from build123d import *

# Parameters (mm, degrees)
F1_DEPTH     = 40.64
F2_SIZE      = 12.7
F3_T1_DEPTH  = 176.0479365306
F3_T3_DEPTH  = 176.0479365306
F3_T5_DEPTH  = 176.0479365306
F3_T7_DEPTH  = 176.0479365306
F3_T9_DEPTH  = 176.0479365306
F3_T11_DEPTH = 176.0479365306
F3_T13_DEPTH = 176.0479365306
F3_T15_DEPTH = 176.0479365306
F3_T17_DEPTH = 176.0479365306
F3_T19_DEPTH = 176.0479365306


# Not quite as in the source:
# - a fillet or chamfer that OpenCascade refuses, or shapes differently, is made with other operations: its cross-section is extruded or revolved along the edge and cut away or added


with BuildPart() as f1:
    # F0 (on Top) → F1 (new body)
    with BuildSketch(Plane.XY):
        Polygon((29.2412366164, 12.8835857291), (16.083875671, 27.6106074452), (-3.2169791099, 31.7913155674), (-21.2890572119, 23.8288216898), (-31.2294390474, 6.7645278386), (-29.2412366164, -12.8835857291), (-16.083875671, -27.6106074452), (3.2169791099, -31.7913155674), (21.2890572119, -23.8288216898), (31.2294390474, -6.7645278386), align=None)
    extrude(amount=F1_DEPTH)

    # F2
    f2_edges = [f1.edges().sort_by_distance(p)[0] for p in [
        (12.253018, -27.810069, 40.64),
        (26.259248, -15.296675, 40.64),
        (30.235338, 3.059529, 40.64),
        (22.662556, 20.247097, 40.64),
        (6.433448, 29.700962, 40.64),
        (-12.253018, 27.810069, 40.64),
        (-26.259248, 15.296675, 40.64),
        (-30.235338, -3.059529, 40.64),
        (-22.662556, -20.247097, 40.64),
        (-6.433448, -29.700962, 40.64),
    ]]
    chamfer(f2_edges, length=F2_SIZE)

    # F3: chamfer of 30.38856 on 10 edges, made by hand

    # F3_s2 → F3_t1 (cut)
    with BuildSketch(Plane(origin=(-86.0289159586, 18.6345004803, 0), x_dir=(0, 0, 1), z_dir=(0.9773351242, -0.2116980278, 0))):
        Polygon((0, 0.001181216), (30.38856, 30.389741216), (0, 30.389741216), align=None)
    extrude(amount=F3_T1_DEPTH, mode=Mode.SUBTRACT)

    # F3_s4 → F3_t3 (cut)
    with BuildSketch(Plane(origin=(8.8619339292, -87.5767384424, 0), x_dir=(0, 0, 1), z_dir=(-0.1006763738, 0.9949192268, 0))):
        Polygon((30.38856, 30.389741216), (0, 0.001181216), (0, 30.389741216), align=None)
    extrude(amount=F3_T3_DEPTH, mode=Mode.SUBTRACT)

    # F3_s6 → F3_t5 (cut)
    with BuildSketch(Plane(origin=(58.645770452, -65.6421556414, 0), x_dir=(0, 0, 1), z_dir=(-0.666247746, 0.7457304747, 0))):
        Polygon((0, 0.001181216), (30.38856, 30.389741216), (0, 30.389741216), align=None)
    extrude(amount=F3_T5_DEPTH, mode=Mode.SUBTRACT)

    # F3_s8 → F3_t7 (cut)
    with BuildSketch(Plane(origin=(86.0289159586, -18.6345004803, 0), x_dir=(0, 0, 1), z_dir=(-0.9773351242, 0.2116980278, 0))):
        Polygon((0, 0.001181216), (30.38856, 30.389741216), (0, 30.389741216), align=None)
    extrude(amount=F3_T7_DEPTH, mode=Mode.SUBTRACT)

    # F3_s10 → F3_t9 (cut)
    with BuildSketch(Plane(origin=(80.5519395843, 35.490900501, 0), x_dir=(0, 0, 1), z_dir=(-0.9151137034, -0.4031958704, 0))):
        Polygon((0, 0.001181216), (30.38856, 30.389741216), (0, 30.389741216), align=None)
    extrude(amount=F3_T9_DEPTH, mode=Mode.SUBTRACT)

    # F3_s12 → F3_t11 (cut)
    with BuildSketch(Plane(origin=(44.3068601486, 76.0599837822, 0), x_dir=(0, 0, 1), z_dir=(-0.5033499514, -0.8640826502, 0))):
        Polygon((0, 0.001181216), (30.38856, 30.389741216), (0, 30.389741216), align=None)
    extrude(amount=F3_T11_DEPTH, mode=Mode.SUBTRACT)

    # F3_s14 → F3_t13 (cut)
    with BuildSketch(Plane(origin=(-8.8619339292, 87.5767384424, 0), x_dir=(0, 0, 1), z_dir=(0.1006763738, -0.9949192268, 0))):
        Polygon((0, 0.001181216), (30.38856, 30.389741216), (0, 30.389741216), align=None)
    extrude(amount=F3_T13_DEPTH, mode=Mode.SUBTRACT)

    # F3_s16 → F3_t15 (cut)
    with BuildSketch(Plane(origin=(-58.645770452, 65.6421556414, 0), x_dir=(0, 0, 1), z_dir=(0.666247746, -0.7457304747, 0))):
        Polygon((0, 0.001181216), (30.38856, 30.389741216), (0, 30.389741216), align=None)
    extrude(amount=F3_T15_DEPTH, mode=Mode.SUBTRACT)

    # F3_s18 → F3_t17 (cut)
    with BuildSketch(Plane(origin=(-80.5519395843, -35.490900501, 0), x_dir=(0, 0, 1), z_dir=(0.9151137034, 0.4031958704, 0))):
        Polygon((0, 0.001181216), (30.38856, 30.389741216), (0, 30.389741216), align=None)
    extrude(amount=F3_T17_DEPTH, mode=Mode.SUBTRACT)

    # F3_s20 → F3_t19 (cut)
    with BuildSketch(Plane(origin=(-44.3068601486, -76.0599837822, 0), x_dir=(0, 0, 1), z_dir=(0.5033499514, 0.8640826502, 0))):
        Polygon((30.38856, 30.389741216), (0, 0.001181216), (0, 30.389741216), align=None)
    extrude(amount=F3_T19_DEPTH, mode=Mode.SUBTRACT)


solid = f1.part
Work out the finished part from the listing and answer in its coordinate system (mm). Coordinates: 2 decimals unless noted, no trailing zeros. Write each loop counter-clockwise with the first axis right and the second up, starting at its lowest first coordinate (ties: lowest second). Pieces come first, ordered by that corner, then holes. Notation, with made-up numbers: (35, -5) - (48, -5) arc R25 cw to (48, 24) - close; hole circle Ø2 at (17, 72). An arc over 180 degrees is marked (long way). One line per question, with ' | ' between items.
1) Find section D-D, the plane z = 21.5. Determine the outline of the cut face in (x, y).
Checks:
outline: (-22.1, 4.79) - (-20.69, -9.12) - (-11.38, -19.53) - (2.28, -22.49) - (15.06, -16.86) - (22.1, -4.79) - (20.69, 9.12) - (11.38, 19.53) - (-2.28, 22.49) - (-15.06, 16.86) - close
2) Consider probe 1 along Z at (x, y) = (-8.5, 13); probe 2 along Z at (x, y) = (24, -11.5); probe 3 along Y at (x, z) = (23.5, 33). Determine where each line is inside the solid, lowest interval first. Write a range as [from, to].
Checks:
probe 1: [15.32, 40.64] | probe 2: [26.53, 31.8] | probe 3: [-9.98, 11.71]
3) Find section A-A, the plane z = 27. Determine the outline of the cut face in (x, y), and give its area (3 significant figures).
Checks:
outline: (-27.75, 6.01) - (-25.98, -11.45) - (-14.29, -24.53) - (2.86, -28.25) - (18.92, -21.17) - (27.75, -6.01) - (25.98, 11.45) - (14.29, 24.53) - (-2.86, 28.25) - (-18.92, 21.17) - close | area: 2,370 mm2
4) Find section C-C, the plane x = 5. Determine the outline of the cut face in (y, z), and give its area (3 significant figures).
Checks:
outline: (-29.67, 29.16) - (-5.6, 7.14) - (-1.08, 4.86) - (2.2, 5.2) - (8.58, 9.45) - (28.76, 29.16) - (17.02, 40.64) - (-17.13, 40.64) - close | area: 1,320 mm2
5) Find section B-B, the plane y = -22. Determine the outline of the cut face in (x, z), and give its area (3 significant figures).
Checks:
outline: (-19.45, 29.16) - (-12.82, 24.21) - (2.23, 21.03) - (19.66, 28.06) - (20.94, 29.16) - (19.66, 30.27) - (2.23, 37.3) - (-12.82, 34.12) - close | area: 392 mm2
6) Flat-ended cylindrical pins translate along their axes: P1, Ø5, axis at x = 20.5, y = -2.5, coming from the -Z side; P2, Ø4, axis at y = 19, z = 18.5, coming from the +X side; P3, Ø4, axis at x = 21.5, y = 14, coming from the +Z side. Find the tip coordinate at first contact, or state that the pin passes through.
Checks:
P1: z = 17.64 | P2: x = 11.06 | P3: z = 34.97
